CAD build for the part. Positions are in the model's coordinates, mm. Face numbers are marked on the shaded views. A direction names the side the tool comes from. Give positions to 0.01 mm unless a question says otherwise; leave off trailing zeros. Write each loop counter-clockwise with the first axis right and the second up, starting at its lowest first coordinate (ties: lowest second). Pieces come first, ordered by that corner, then holes. Notation, with made-up numbers: (67.25, 84.25) - (86.25, 84.25) arc R24 ccw to (86.25, 113.25) - close; hole circle Ø5 at (37.5, 68). An arc over 180 degrees is marked (long way). Answer as a JSON object with one key per item and string values.
from build123d import *

# Parameters (mm, degrees)
F1_DEPTH  = 10.3
F2_R      = 1.55
F2_R_2    = 2.5
F2_W      = 18.2711938396
F2_H      = 41.0630945116
F2_W_2    = 3.7480126619
F2_H_2    = 6.4359663129
F3_DEPTH  = 10.3
F4_R      = 3
F5_R      = 5
F6_R      = 4.25
F7_DEPTH  = 5.8
F8_R      = 1.55
F9_DEPTH  = 25
F11_DEPTH = 4


with BuildPart() as f1:
    # F0 (on Top) → F1 (new body)
    with BuildSketch(Plane.XY):
        with BuildLine():
            Line((23, -15.75), (23, 35.75))
            Line((23, 35.75), (-23, 35.75))
            Line((-23, 35.75), (-23, -15.75))
            ThreePointArc((-23, -15.75), (0, -35.5223387435), (23, -15.75))
        make_face()
    extrude(amount=F1_DEPTH)

    # F2 (on face) → F3 (cut, through all)
    with BuildSketch(Plane.XY.offset(10.3)):
        with Locations((11, 28.55)):
            Circle(F2_R)
        with Locations((-8.75, 28.55)):
            Circle(F2_R)
        with Locations((11, 5.7171783878)):
            Circle(F2_R)
        with Locations((18, 25.75)):
            Circle(F2_R_2)
        with Locations((18, -14.25)):
            Circle(F2_R_2)
        with Locations((-18, 5.8170498922)):
            Circle(F2_R_2)
        with Locations((-3.1221020035, -2.9017189518)):
            Rectangle(F2_W, F2_H)
        Polygon((-12.2576989233, 17.6298283041), (6.0134949163, 17.6298283041), (6.0134949163, 18.8598968089), (-12.2576989233, 18.8598968089), (-13.8854337856, 18.8598968089), (-13.8854337856, 29.3140336871), (-15.5863631517, 29.3140336871), (-19.2519873381, 29.3140336871), (-23, 29.3140336871), (-23, 27.7502387762), (-17.4777284265, 27.7502387762), (-17.4777284265, 17.6298283041), (-15.5863631517, 17.6298283041), align=None)
        with BuildLine():
            ThreePointArc((-12.2576989233, -23.4332662076), (-3.1221020035, -28.5924931443), (6.0134949163, -23.4332662076))
            Line((6.0134949163, -23.4332662076), (-12.2576989233, -23.4332662076))
        make_face()
        with Locations((-21.125993669, 32.5320168436)):
            Rectangle(F2_W_2, F2_H_2)
    extrude(amount=-F3_DEPTH, mode=Mode.SUBTRACT)

    # F4
    f4_edges = [f1.edges().sort_by_distance(p)[0] for p in [
        (-12.257699, 17.629828, 5.15),
    ]]
    fillet(f4_edges, radius=F4_R)

    # F5
    f5_edges = [f1.edges().sort_by_distance(p)[0] for p in [
        (-19.251987, 35.75, 5.15),
        (23, 35.75, 5.15),
        (-12.257699, -23.433266, 5.15),
        (6.013495, -23.433266, 5.15),
        (6.013495, 18.859897, 5.15),
    ]]
    fillet(f5_edges, radius=F5_R)

    # F6 (on face) → F7 (cut)
    with BuildSketch(Plane.XY.offset(10.3)):
        with Locations((18, 25.75)):
            Circle(F6_R)
        with Locations((-18, 5.8170498922)):
            Circle(F6_R)
        with Locations((18, -14.25)):
            Circle(F6_R)
    extrude(amount=-F7_DEPTH, mode=Mode.SUBTRACT)

    # F8 (on face) → F9 (cut)
    with BuildSketch(Plane(origin=(-23, 0, 0), x_dir=(0, -1, 0), z_dir=(-1, 0, 0))):
        with Locations((-23.8586217165, 5.15)):
            Circle(F8_R)
    extrude(amount=-F9_DEPTH, mode=Mode.SUBTRACT)

    # F10 (on face) → F11 (cut)
    with BuildSketch(Plane(origin=(0, 0, 0), x_dir=(1, 0, 0), z_dir=(0, 0, -1))):
        Polygon((11.0856638946, -25.1447107273), (8.09376493, -26.7731682547), (8.0081010353, -30.1784575274), (10.9143361054, -31.9552892727), (13.90623507, -30.3268317453), (13.9918989647, -26.9215424726), align=None)
        Polygon((-8.7919851376, -25.1438921653), (-11.7207684817, -26.8833062784), (-11.6787833441, -30.2894141131), (-8.7080148624, -31.9561078347), (-5.7792315183, -30.2166937216), (-5.8212166559, -26.8105858869), align=None)
        Polygon((10.8521251413, -2.3140230343), (7.9788435816, -4.1436640952), (8.1267184402, -7.5468194487), (11.1478748587, -9.1203337412), (14.0211564184, -7.2906926803), (13.8732815598, -3.8875373269), align=None)
    extrude(amount=-F11_DEPTH, mode=Mode.SUBTRACT)


solid = f1.part
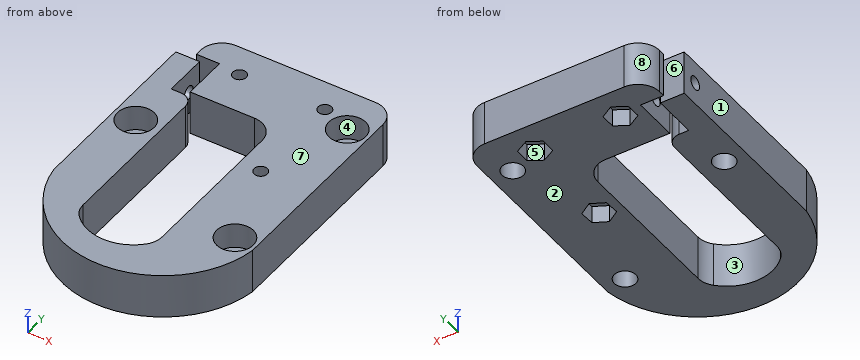
(1) Saw through at B-B, the plane x = 19.5. Give the cut face in (y, z), and give its area (3 significant figures).
Answer key:
{"outline": "(-24.95, 0) - (-16.25, 0) - (-16.25, 4.5) - (-18.23, 4.5) - (-18.23, 10.3) - (-24.95, 10.3) - close; (-12.25, 0) - (23.75, 0) - (23.75, 4.5) - (21.77, 4.5) - (21.77, 10.3) - (-10.27, 10.3) - (-10.27, 4.5) - (-12.25, 4.5) - close; (27.75, 0) - (35.52, 0) - (35.52, 10.3) - (29.73, 10.3) - (29.73, 4.5) - (27.75, 4.5) - close", "area": "495 mm²"}
(2) Probe L1, parallel to Y at x = 11, z = 5; L2, parallel to Y at x = 12, z = 6.25; L3, parallel to X at y = 1.5, z = 9. List the from-to ranges inside material, lowest first. Write a range as [from, to].
Answer key:
{"L1": "y = [-32.76, 4.17], [7.27, 27], [30.1, 35.75]", "L2": "y = [-32.19, 4.53], [6.9, 27.37], [29.73, 35.75]", "L3": "x = [-23, -12.26], [6.01, 23]"}
(3) Pull direction Y, two halves, no side cores. Call the marked faces 6, 7 and 8: pulls with the +Y half, pulls with the -Y half, needs draft (parallel to the pull), parting line crosses it, or undercut.
Answer key:
{"face 6": "undercut", "face 7": "needs draft", "face 8": "pulls with the +Y half"}
(4) 3-axis set-ups, long thin cutter, end or side, ignore diameter. For the marked faces 1, 2, 3, 4 and 5: which of +Z, -Z, +X, -X, +Y, -Y reach the whole face in a straight line?
Answer key:
{"face 1": "+Z, -Z, -X, +Y, -Y", "face 2": "-Z, +X, -X, +Y, -Y", "face 3": "+Z, -Z", "face 4": "+Z", "face 5": "-Z"}
(5) Flat gauge pins, fed straight in: P1, Ø6, axis at x = -10.5, z = 6.5, coming from the -Y side; P2, Ø3, axis at x = -8.75, y = 28.55, coming from the +Z side; P3, Ø6, axis at x = 18, y = -14.25, coming from the +Z side; P4, Ø3, axis at x = -7, z = 6, coming from the -Y side. Where does each tip first touch, or does it go through?
Answer key:
{"P1": "stops at y = -34.28", "P2": "passes through", "P3": "stops at z = 4.5", "P4": "stops at y = -34.86"}
(6) Saw through at C-C, the plane y = 16. Give the cut face in (x, z), and give its area (3 significant figures).
Answer key:
{"outline": "(-23, 0) - (-12.59, 0) - (-12.59, 10.3) - (-23, 10.3) - close; (5.53, 0) - (23, 0) - (23, 10.3) - (5.53, 10.3) - close", "area": "287 mm²"}
(7) Saw through at A-A, the plane z = 9. Give the cut face in (x, y), and give its area (3 significant figures).
Answer key:
{"outline": "(-23, -15.75) arc R23.26 ccw to (23, -15.75) - (23, 30.75) arc R5 ccw to (18, 35.75) - (-14.25, 35.75) arc R5 ccw to (-19.25, 30.75) - (-19.25, 29.31) - (-13.89, 29.31) - (-13.89, 18.86) - (1.01, 18.86) arc R5 cw to (6.01, 13.86) - (6.01, -21.8) arc R5 cw to (4.66, -25.22) arc R10.67 cw to (-10.91, -25.22) arc R5 cw to (-12.26, -21.8) - (-12.26, 14.63) arc R3 ccw to (-15.26, 17.63) - (-17.48, 17.63) - (-17.48, 27.75) - (-23, 27.75) - close; hole circle Ø8.5 at (-18, 5.82); hole circle Ø3.1 at (-8.75, 28.55); hole circle Ø3.1 at (11, 5.72); hole circle Ø3.1 at (11, 28.55); hole circle Ø8.5 at (18, -14.25); hole circle Ø8.5 at (18, 25.75)", "area": "1,940 mm²"}
(8) Saw through at D-D, the plane z = 1. State how many separate pieces and enclosed holes the cut face has, and give its area (3 significant figures).
Answer key:
{"separate pieces": "1", "enclosed holes": "6", "area": "1,990 mm²"}
